Can you work these out from the drawing? Everything is in mm from the part's minimum corner. A direction names the side the tool comes from. Coordinates: 2 decimals unless noted, no trailing zeros. Order: outer loops, then holes, each group sorted by start corner. A loop starts at its lowest first (then second) coordinate and runs counter-clockwise, first axis right, second up. Notation, with made-up numbers: M 70,84.5 L 106,84.5 A29 cw 106,105.5 Z; hole C 9.5,17.25 d6. An arc over 180 degrees is marked long. Answer as a JSON object with one key per item and string values.
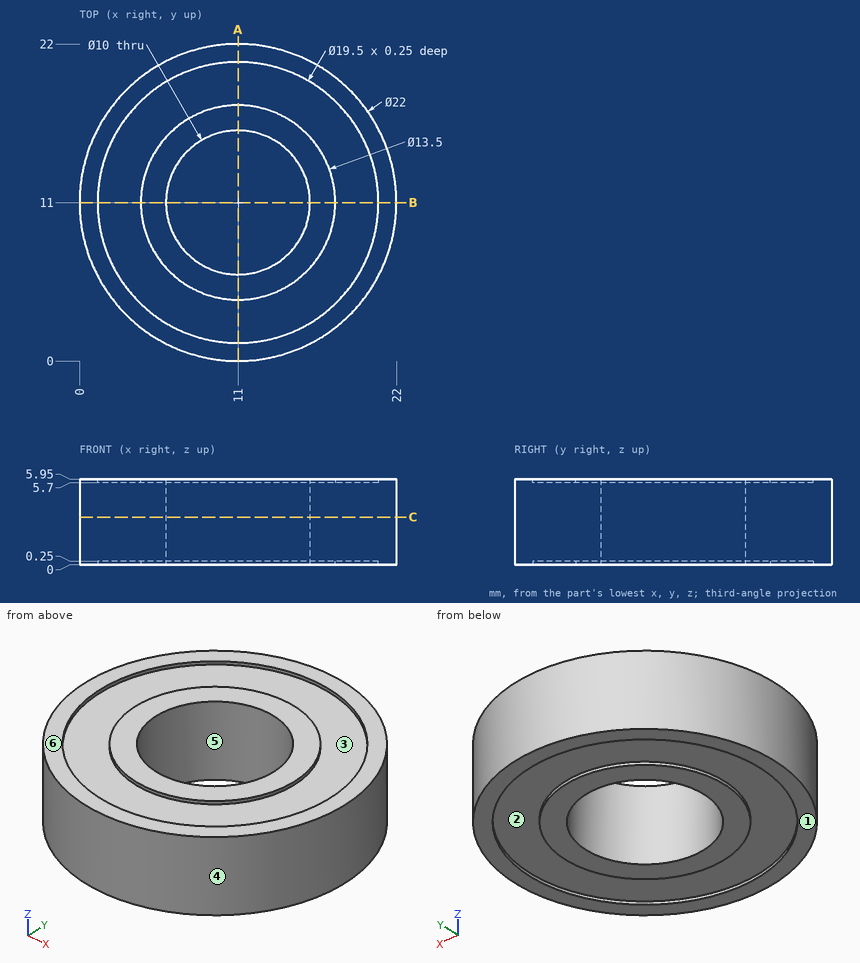
Item 1: I want a section at A-A, the plane x = 11. Write out the boundary of the cut face in (y, z), plus the area to 3 significant figures.
Answers follow:
{"outline": "M 0,0 L 1.25,0 L 1.25,0.25 L 4.25,0.25 L 4.25,0 L 6,0 L 6,5.95 L 4.25,5.95 L 4.25,5.7 L 1.25,5.7 L 1.25,5.95 L 0,5.95 Z; M 16,0 L 17.75,0 L 17.75,0.25 L 20.75,0.25 L 20.75,0 L 22,0 L 22,5.95 L 20.75,5.95 L 20.75,5.7 L 17.75,5.7 L 17.75,5.95 L 16,5.95 Z", "area": "68.4 mm^2"}
Item 2: I want a section at C-C, the plane z = 3.3. Write out the boundary of the cut face in (x, y), plus the area to 3 significant figures.
Answers follow:
{"outline": "C 11,11 d22; hole C 11,11 d10", "area": "302 mm^2"}
Item 3: Please list where these lines run through material, in increasing order: line 1 (Y direction, x = 11, z = 5.85); line 2 (Y direction, x = 11, z = 4.1); line 3 (X direction, y = 10.75, z = 4.8).
Answers follow:
{"line 1": "y = 0 to 1.25, 4.25 to 6, 16 to 17.75, 20.75 to 22", "line 2": "y = 0 to 6, 16 to 22", "line 3": "x = 0 to 6.01, 15.99 to 22"}
Item 4: If we mould it in two halves opening along X, with no side actions, what happens to the marked faces 3, 4, 5 and 6? For each: pulls with the +X half, pulls with the -X half, needs draft (parallel to the pull), parting line crosses it, or undercut.
Answers follow:
{"face 3": "undercut", "face 4": "parting line crosses it", "face 5": "undercut", "face 6": "needs draft"}
Item 5: I'm going to push flat-ended pins straight in: pin 1 (1.5 mm diameter, centred on x = 4.5, z = 0.5, fed in from +Y); pin 2 (8 mm diameter, centred on x = 11, y = 11, fed in from -Z). Where does each tip first touch, or does it pass through?
Answers follow:
{"pin 1": "stops at y = 20.38", "pin 2": "passes through"}
Item 6: Which directions (+Z, -Z, +X, -X, +Y, -Y) give clear straight access to the entire face, cutting with the end or side of a thin tool? Please do the marked faces 1 and 2.
Answers follow:
{"face 1": "-Z, +X, -X, +Y, -Y", "face 2": "-Z"}
